Autodesk Inventor part; units mm, degrees
ref_plane "YZ Plane" through (0, 0, 0) normal (1, 0, 0) x (0, 1, 0)
ref_plane "XZ Plane" through (0, 0, 0) normal (0, 1, 0) x (-1, 0, 0)
ref_plane "XY Plane" through (0, 0, 0) normal (0, 0, 1) x (1, 0, 0)
ref_plane "Arbeitsebene1" through (15, 0, 0) normal (-1, 0, 0) x (0, 1, 0)
sketch "Skizze1" plane through (15, 0, 0) normal (-1, 0, 0) x (0, 1, 0)
  line L0 (32.6031, 0.5) -> (30.7237, 0.5)
  line L1 (30.7237, 4.25) -> (32.6031, 4.25)
  line L2 (30.7237, 0.5) -> (30.7237, 4.25)
  line L3 (32.6031, 0.5) -> (30.7237, 0.5)
  line L4 (30.7237, 4.7) -> (32.6031, 4.7)
  line L5 (30.7237, 0.5) -> (30.7237, 4.25)
  line L6 (30, 0.5) -> (32, 0.5)
  line L7 (30, 0.55) -> (30, 0.5)
  line L8 (32, 0.5) -> (32, 0.55)
  line L9 (32, 0.5) -> (32, 16.1)
  line L10 (52, 0.5) -> (52, 16.1)
  line L11 (42, 19.32) -> (42, -3.22)
  line L12 (32.6031, 0.5) -> (27, 0.5)
  line L13 (27, 0.5) -> (27, -2.5)
  line L14 (27, -2.5) -> (35.6031, -2.5)
  line L15 (35.6031, -2.5) -> (35.6031, 5.25)
  line L16 (35.6031, 5.25) -> (34.1031, 5.25)
  line L17 (32.6031, 0.5) -> (32.6031, 0.2)
  line L18 (32.6031, 0.2) -> (27, 0.2)
  line L19 (32, 0.55) -> (30, 0.55)
  line L20 (32.1031, 0.5) -> (32.0412, 0.2)
  line L21 (27, -2.5) -> (32, -2.5)
  line L22 (32, -2.5) -> (32, -10.5)
  line L23 (32, -10.5) -> (27, -10.5)
  line L24 (27, -10.5) -> (27, -2.5)
  line L25 (34.1031, 5.25) -> (32.307, 3.9176)
  line L26 (32.307, 3.9176) -> (32.1031, 0.5)
  point P0 (0, 0)
  point P1 (32, -2.5)
  point P2 (30.7237, 0.55)
  point P3 (32, 4.25)
  dimension "d1" = 3
  dimension "d3" = 1
  dimension "d11" = 0.5
  dimension "d13" = 15
  dimension "d14" = 8
  dimension "d15" = 10
  dimension "d37" = 0.3
  dimension "d38" = 6.3969
revolve "Umdrehung1" add sketch "Skizze1" angle 360 about axis through (15, 42, -19.32) along (0, 0, 1) contours L17 L18 L20 L0 | L0 L26 L25 L16 L15 L14 L13 L18 L17
sketch "Skizze2" plane through (0, 0, 0) normal (0, 1, 0) x (-1, 0, 0)
  spline S0 degree 3 poles (-15, -4.25) (-12.1304, -4.4784) (-9.2732, -4.7067) (-7.1109, -4.9351) (-6.8554, -4.962) (-6.6095, -4.989) (-6.3738, -5.016) knots 0 0 0 0 0.7174 0.7174 0.7174 0.802142 0.802142 0.802142 0.802142
  spline S1 degree 3 poles (-14.5016, -1.0897) (-11.6314, -1.3183) (-8.8183, -1.5469) (-6.7355, -1.7755) (-6.2054, -1.8336) (-5.7215, -1.8918) (-5.2918, -1.95) knots 0.041547 0.041547 0.041547 0.041547 0.759706 0.759706 0.759706 0.942478 0.942478 0.942478 0.942478
  circle A0 centre (-15, -2.8138) radius 1.4
  line L0 (-15, 1.0048) -> (-15, -6.0288)
  point P0 (0, 0)
  dimension "d5" = 2.8
extrude "Extrusion1" cut sketch "Skizze2" along normal up to surface
pattern_circular "Runde Anordnung1" count 3 over 360 about axis through (15, 42, 1.15) along (0, 0, -1) of "Extrusion1"
chamfer "Fase1" distance 1 angle 45 1 edges at (15, 48.3969, 2.5)
sketch "Skizze6" plane through (15, 42, 2.5) normal (0, 0, 1) x (1, 0, 0)
  circle A0 centre (0, 0) radius 15
  circle A1 centre (0, 0) radius 7.3969
  circle A2 centre (0, 0) radius 13.15
  circle A3 centre (0, 0) radius 9.5
  point P0 (-15, -42)
  dimension "d31" = 26.3
  dimension "d39" = 19
extrude "Extrusion4" cut sketch "Skizze6" against normal blind 1 contours A2
properties part number "30_Linear_Stage_NEMA11_baseholder_bayonetmount_objective_rms_metaladapter"
Verification items for the finished model (mm, model axes). A direction names the side the tool comes from. Round coordinates to 2 decimals unless told otherwise and drop trailing zeros. Loops run counter-clockwise (first coordinate to the right, second up) from the corner with the lowest first, then second, coordinate; pieces in that order, holes last. Notation, with made-up numbers: (37.25, 13.5) -> (83.25, 13.5) arc R23 ccw to (83.25, 31.5) -> close; hole circle Ø9 at (23, 12.5). An arc over 180 degrees is marked (long way). Answer as a JSON object with one key per item and string values.
Q1. Draft check along Y on faces 6 (the flat face through (19, 33, 1.5)), 7 (the flat face through (1.7, 42.1, 2.5)), 8 (the cylindrical face through (14.72, 48.39, -1.92)), 9 (the conical face through (21.59, 49.19, -2.94)). Enter one of: pulls with the +Y half, pulls with the -Y half, needs draft (parallel to the pull), parting line crosses it, or undercut.
Data:
{"face 6": "undercut", "face 7": "needs draft", "face 8": "undercut", "face 9": "parting line crosses it"}
Q2. Scan lines: line 1 (Z direction, x = 7.5, y = 50.5); line 2 (Z direction, x = 16, y = 35.5); line 3 (X direction, y = 40.25, z = 0). Record each from-to range of solid material in increasing order. Write a range as from..to.
Data:
{"line 1": "z = -0.2..1.5", "line 2": "z = -5.25..-3.79, -1.83..1.68", "line 3": "x = 0.1..8.85, 21.15..29.9"}
Q3. Section check B-B (z = 0.5). Record the boundary of the cut face in (x, y), then the cut area to 3 significant figures.
Data:
{"outline": "circle Ø30 at (15, 42); hole circle Ø12.79 at (15, 42)", "area": "578 mm2"}
Q4. Access from +Z, -Z, +X, -X, +Y, -Y to the whole of each face (thin tool, end or side, straight path). Record for faces 1 (the cylindrical face through (8.34, 46.59, -1.57)), 2 (the cylindrical face through (15.303, 33.933, -1.447)), 3 (the flat face through (12, 32, -0.2)), 4 (the cylindrical face through (8, 48.42, 2.01)), 5 (the cylindrical face through (15.66, 56.985, 1.169)).
Data:
{"face 1": "none", "face 2": "-Y", "face 3": "-Z", "face 4": "+Z", "face 5": "+Z, -Z"}
Q5. Go/stop test with flat-tipped pins: P1, Ø8, axis at x = 13, y = 39.5, coming from the +Z side; P2, Ø12, axis at x = 12, y = 31, coming from the -Z side; P3, Ø2, axis at x = 15, z = -2.81, coming from the -Y side. Record where each tip stops, or that it passes through.
Data:
{"P1": "stops at z = 2.3", "P2": "stops at z = -5.25", "P3": "stops at y = 48.32"}
Q6. Section check C-C (x = 15). State how many separate pieces and enclosed holes the cut face has, then the cut area to 3 significant figures.
Data:
{"separate pieces": "3", "enclosed holes": "0", "area": "60.5 mm2"}
Q7. Section check D-D (y = 30.75). Record the boundary of the cut face in (x, z), then the cut area to 3 significant figures.
Data:
{"outline": "(5.08, -0.2) -> (24.92, -0.2) -> (24.92, 2.5) -> (21.81, 2.5) -> (21.81, 1.5) -> (8.19, 1.5) -> (8.19, 2.5) -> (5.08, 2.5) -> close", "area": "40.0 mm2"}
Q8. Section check A-A (y = 42). Record the boundary of the cut face in (x, z), then the cut area to 3 significant figures.
Data:
{"outline": "(0, -0.2) -> (5.04, -0.2) -> (5.1, -0.5) -> (5.31, -3.92) -> (7.1, -5.25) -> (8.6, -5.25) -> (8.6, 1.5) -> (7.6, 2.5) -> (5.5, 2.5) -> (5.5, 1.5) -> (1.85, 1.5) -> (1.85, 2.5) -> (0, 2.5) -> close; (21.4, -5.25) -> (22.9, -5.25) -> (24.69, -3.92) -> (24.9, -0.5) -> (24.96, -0.2) -> (30, -0.2) -> (30, 2.5) -> (28.15, 2.5) -> (28.15, 1.5) -> (24.5, 1.5) -> (24.5, 2.5) -> (22.4, 2.5) -> (21.4, 1.5) -> close", "area": "69.9 mm2"}
